from build123d import *

# Parameters (mm, degrees)
SKETCH1_W           = 10
SKETCH1_H           = 36
BOSS_EXTRUDE2_DEPTH = 4
SKETCH5_R           = 3
BOSS_EXTRUDE3_DEPTH = 10
SKETCH6_R           = 2.5
BOSS_EXTRUDE4_DEPTH = 10
SKETCH9_R           = 1.5
CUT_EXTRUDE2_DEPTH  = 10
SKETCH10_W          = 5
SKETCH10_H          = 8
CUT_EXTRUDE3_DEPTH  = 4
SKETCH11_W          = 4
SKETCH11_H          = 0.5
BOSS_EXTRUDE6_DEPTH = 5
BOSS_EXTRUDE7_DEPTH = 10
SKETCH7_R           = 1.5
CUT_EXTRUDE4_DEPTH  = 10
SKETCH14_W          = 10
SKETCH14_H          = 4
BOSS_EXTRUDE8_DEPTH = 15
FILLET2_R           = 2
CHAMFER1_SIZE       = 10
CHAMFER1_SIZE2      = 3.639702343


with BuildPart() as part:
    # Sketch1 → Boss-Extrude2 (new body)
    with BuildSketch(Plane(origin=(0, 0, 0), x_dir=(1, 0, 0), z_dir=(0, 1, 0))):
        Rectangle(SKETCH1_W, SKETCH1_H)
    extrude(amount=BOSS_EXTRUDE2_DEPTH)

    # Sketch5 → Boss-Extrude3 (add)
    with BuildSketch(Plane(origin=(5, 0, 0), x_dir=(0, 0, -1), z_dir=(1, 0, 0))):
        with Locations((-18, 2)):
            Circle(SKETCH5_R)
    extrude(amount=-BOSS_EXTRUDE3_DEPTH)

    # Sketch6 → Boss-Extrude4 (add)
    with BuildSketch(Plane(origin=(5, 0, 0), x_dir=(0, 0, -1), z_dir=(1, 0, 0))):
        with Locations((18, 2)):
            Circle(SKETCH6_R)
    extrude(amount=-BOSS_EXTRUDE4_DEPTH)

    # Sketch9 → Cut-Extrude2 (cut)
    with BuildSketch(Plane(origin=(5, 0, 0), x_dir=(0, 0, -1), z_dir=(1, 0, 0))):
        with Locations((18, 2)):
            Circle(SKETCH9_R)
    extrude(amount=-CUT_EXTRUDE2_DEPTH, mode=Mode.SUBTRACT)

    # Sketch10 → Cut-Extrude3 (cut)
    with BuildSketch(Plane(origin=(0, 4, 0), x_dir=(1, 0, 0), z_dir=(0, 1, 0))):
        with Locations((0, 16.5)):
            Rectangle(SKETCH10_W, SKETCH10_H)
    extrude(amount=-CUT_EXTRUDE3_DEPTH, mode=Mode.SUBTRACT)

    # Sketch11 → Boss-Extrude6 (add)
    with BuildSketch(Plane.ZY.offset(-2.5)):
        with Locations((-18, 2)):
            Rectangle(SKETCH11_W, SKETCH11_H)
    extrude(amount=BOSS_EXTRUDE6_DEPTH)

    # Sketch13 → Boss-Extrude7 (add)
    with BuildSketch(Plane(origin=(5, 0, 0), x_dir=(0, 0, -1), z_dir=(1, 0, 0))):
        Polygon((-19.282983434, 4.711817381), (-71.244507661, -25.288182619), (-69.244507661, -28.752284234), (-17.282983434, 1.247715766), align=None)
    extrude(amount=-BOSS_EXTRUDE7_DEPTH)

    # Sketch7 → Cut-Extrude4 (cut)
    with BuildSketch(Plane(origin=(5, 0, 0), x_dir=(0, 0, -1), z_dir=(1, 0, 0))):
        with Locations((-18, 2)):
            Circle(SKETCH7_R)
    extrude(amount=-CUT_EXTRUDE4_DEPTH, mode=Mode.SUBTRACT)

    # Sketch14 → Boss-Extrude8 (add)
    with BuildSketch(Plane(origin=(0, 11.883639793, 6.861022633), x_dir=(1, 0, 0), z_dir=(0, 0.8660254037844415, 0.49999999999999506))):
        with Locations((0, -72.343644824)):
            Rectangle(SKETCH14_W, SKETCH14_H)
    extrude(amount=BOSS_EXTRUDE8_DEPTH)

    # Fillet2
    fillet2_edges = [part.edges().sort_by_distance(p)[0] for p in [
        (0, -28.752284234, 69.244507661),
    ]]
    fillet(fillet2_edges, radius=FILLET2_R)

    # Chamfer1
    chamfer1_edges = [part.edges().sort_by_distance(p)[0] for p in [
        (0, -10.297801562, 75.280406046),
    ]]
    chamfer1_side = [part.faces().sort_by_distance(p)[0] for p in [
        (0, -16.792992091, 71.530406046),
    ]]
    chamfer(chamfer1_edges, length=CHAMFER1_SIZE, length2=CHAMFER1_SIZE2, reference=chamfer1_side[0])


solid = part.part
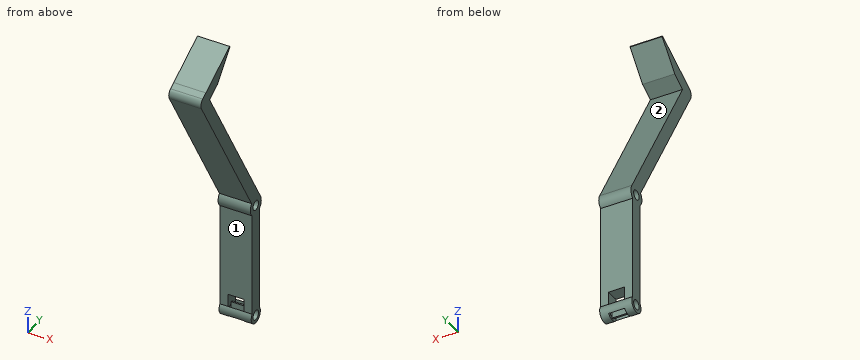
Can you work these out from the model? Positions are in its coordinate system, mm. Face numbers are marked on the shaded views. A direction names the side the tool comes from. Coordinates: 2 decimals unless noted, no trailing zeros. Loops run counter-clockwise (first coordinate to the right, second up) from the corner with the lowest first, then second, coordinate; pieces in that order, holes last. Notation, with made-up numbers: M 64,-2.5 L 116,-2.5 A26 cw 116,19.5 Z; hole C -28.75,-22 d10. An arc over 180 degrees is marked long. Return JSON: item names as keys, results as strings. Group by question number.
Item 1: Imagine slicing it at D-D (x = 3.75). Please give me the cut outline in (y, z), and give its area (3 significant figures).
Item 2: Imagine slicing it at B-B (x = -1). Please give me the cut outline in (y, z), and give its area (3 significant figures).
Item 3: On a 3-axis mill with a long thin cutter (end or side, diameter ignored), from which of +Z, -Z, +X, -X, +Y, -Y can I reach the whole of each face in a straight line? I mean the marked faces 1 and 2. Say none if no direction works.
Item 4: If I drill on L1, parallel to Y at x = 3.25, z = -18; L2, parallel to Z at x = -4, y = -14; L3, parallel to Y at x = 1.5, z = 18, over which ranges is the centre line in solid material (lowest first)? Write a range as from..to.
Item 5: I'm going to push flat-ended pins straight in: pin 1 Ø1.5 at (x, z) = (-1, -1.5) entering from -Y; pin 2 Ø0.9 at (x, z) = (-1, -18.5) entering from -Y; pin 3 Ø0.9 at (x, z) = (-1, -17.5) entering from +Y. Where does each tip first touch, or does it pass through?
Item 6: Imagine slicing it at A-A (z = -18). Please give me the cut outline in (x, y).
Item 7: Imagine slicing it at C-C (z = 18). Please give me the cut outline in (x, y), and give its area (3 significant figures).
Verdict:
{
 "1": {"outline": "M -27.75,67.51 L -0.29,19.94 A3 ccw 0,15.76 L 0,-16.5 A2.5 ccw long 4,-16.5 L 4,15.76 A3 ccw 4.47,19.71 L -23.29,67.78 L -18.96,70.28 L -12.12,78.43 L -12.3,78.74 L -27.02,70.24 A2 ccw Z; hole C 2,-18 d3; hole C 2,18 d3", "area": "428 mm^2"},
 "2": {"outline": "M -27.75,67.51 L -0.29,19.94 A3 ccw 0,15.76 L 0,-12.5 L 4,-12.5 L 4,15.76 A3 ccw 4.47,19.71 L -23.29,67.78 L -18.96,70.28 L -12.12,78.43 L -12.3,78.74 L -27.02,70.24 A2 ccw Z; M 0,-19.5 L 0,-16.5 A2.5 ccw Z; M 1.75,-20 L 2.25,-20 L 2.25,-16 L 1.75,-16 Z; M 4,-19.5 A2.5 ccw 4,-16.5 Z; hole C 2,18 d3", "area": "406 mm^2"},
 "3": {"face 1": "+X, -X, -Y", "face 2": "+X, -X, +Y"},
 "4": {"L1": "y = -0.5..0.5, 3.5..4.5", "L2": "z = 43.69..51.69, 76.19..77.76", "L3": "y = -1..0.5, 3.5..5"},
 "5": {"pin 1": "stops at y = 0", "pin 2": "stops at y = -0.5", "pin 3": "stops at y = 4.5"},
 "6": {"outline": "M -5,-0.5 L 5,-0.5 L 5,0.5 L 2.5,0.5 L 2.5,0 L -2.5,0 L -2.5,0.5 L -5,0.5 Z; M -5,3.5 L -2.5,3.5 L -2.5,4 L 2.5,4 L 2.5,3.5 L 5,3.5 L 5,4.5 L -5,4.5 Z; M -2.5,1.75 L 2.5,1.75 L 2.5,2.25 L -2.5,2.25 Z"},
 "7": {"outline": "M -5,-1 L 5,-1 L 5,0.5 L -5,0.5 Z; M -5,3.5 L 5,3.5 L 5,5 L -5,5 Z", "area": "30.0 mm^2"}
}
